```python
from build123d import *

# Parameters (mm, degrees)
SKETCH1_W           = 200
SKETCH1_H           = 150
BOSS_EXTRUDE1_DEPTH = 4
FILLET1_R           = 2
FILLET2_R           = 2
FILLET3_R           = 2
FILLET4_R           = 2
SKETCH2_W           = 8
SKETCH2_H           = 30
BOSS_EXTRUDE2_DEPTH = 4
FILLET5_R           = 2


# Some blends are built 0.0001 mm under size
with BuildPart() as part:
    # Sketch1 → Boss-Extrude1 (new body)
    with BuildSketch(Plane(origin=(0, 0, 0), x_dir=(1, 0, 0), z_dir=(0, 1, 0))):
        with Locations((-106.41025641, 19.711538462)):
            Rectangle(SKETCH1_W, SKETCH1_H)
    extrude(amount=BOSS_EXTRUDE1_DEPTH)

    # Fillet1
    fillet1_edges = [part.edges().sort_by_distance(p)[0] for p in [
        (-206.41025641, 4, -19.711538462),
        (-106.41025641, 4, -94.711538462),
    ]]
    fillet(fillet1_edges, radius=FILLET1_R)

    # Fillet2
    fillet2_edges = [part.edges().sort_by_distance(p)[0] for p in [
        (-105.41025641, 4, 55.288461538),
        (-206.41025641, 1, 55.288461538),
        (-205.824469973, 3.414213562, 55.288461538),
    ]]
    fillet(fillet2_edges, radius=FILLET2_R)

    # Fillet3
    fillet3_edges = [part.edges().sort_by_distance(p)[0] for p in [
        (-6.41025641, 1, -94.711538462),
        (-6.41025641, 3.414213562, -94.125752024),
        (-6.41025641, 1, 55.288461538),
        (-6.41025641, 4, -19.711538462),
        (-6.41025641, 3.414213562, 54.702675101),
    ]]
    fillet(fillet3_edges, radius=FILLET3_R)

    # Fillet4
    # the kernel refuses this fillet: 2 mm, written as the material it takes off along each edge
    with BuildSketch(Plane(origin=(-204.41025641, 2, -92.711538462), x_dir=(-1, 0, 0), z_dir=(0, 0, -1))) as fillet4_piece_1_section:
        Polygon((0, 0), (FILLET4_R, 0), (FILLET4_R, FILLET4_R), (0, FILLET4_R), align=None)
    fillet4_piece_1 = extrude(amount=FILLET4_R, mode=Mode.PRIVATE)
    fillet4_piece_1 = fillet4_piece_1 - Plane(origin=(-204.41025641, 2, -92.711538462), x_dir=(0.7071067811865475, -0.7071067811865475, 0), z_dir=(0, 0, -1)) * Sphere(FILLET4_R, mode=Mode.PRIVATE)
    add(fillet4_piece_1, mode=Mode.SUBTRACT)
    with BuildSketch(Plane(origin=(-206.41025641, -5, -94.711538462), x_dir=(1, 0, 0), z_dir=(0, 1, 0))) as fillet4_piece_2:
        with BuildLine():
            CenterArc((FILLET4_R, -FILLET4_R), FILLET4_R, 90, 90)
            Line((0, -FILLET4_R), (0, 0))
            Line((0, 0), (FILLET4_R, 0))
        make_face()
    extrude(amount=7, mode=Mode.SUBTRACT)

    # Sketch2 → Boss-Extrude2 (add)
    with BuildSketch(Plane(origin=(0, 4, 0), x_dir=(1, 0, 0), z_dir=(0, 1, 0))):
        with Locations((-6.865890451, 22.549136896)):
            Rectangle(SKETCH2_W, SKETCH2_H)
    extrude(amount=-BOSS_EXTRUDE2_DEPTH)

    # Fillet5
    fillet5_edges = [part.edges().sort_by_distance(p)[0] for p in [
        (-4.638073431, 0, -37.549136896),
    ]]
    fillet(fillet5_edges, radius=FILLET5_R)
    fillet5_2_edges = [part.edges().sort_by_distance(p)[0] for p in [
        (-2.865890451, 0, -21.549136896),
    ]]
    fillet(fillet5_2_edges, radius=FILLET5_R)
    fillet5_3_edges = [part.edges().sort_by_distance(p)[0] for p in [
        (-5.638073431, 0, -7.549136896),
    ]]
    fillet(fillet5_3_edges, radius=FILLET5_R)
    fillet5_4_edges = [part.edges().sort_by_distance(p)[0] for p in [
        (-6.638073431, 4, -37.549136896),
    ]]
    fillet(fillet5_4_edges, radius=FILLET5_R - 0.0001)  # a hair under: the kernel refuses the full size


solid = part.part
```
Can you work these out from the model? Positions are in its coordinate system, mm. Give positions to 0.01 mm unless a question says otherwise; leave off trailing zeros. Loops run counter-clockwise (first coordinate to the right, second up) from the corner with the lowest first, then second, coordinate; pieces in that order, holes last. Notation, with made-up numbers: M 8.5,-16 L 66.5,-16 A9 cw 66.5,-5 Z; hole C 61.5,80 d7. An arc over 180 degrees is marked long. Answer in a Markdown table with one row per item.
1. Suppose I cut it at A-A on z = -78. Write out the boundary of the cut face in (x, y), plus the area to 3 significant figures.
Taken from the geometry:
| item | result |
|---|---|
| outline | M -206.41,0 L -6.41,0 L -6.41,2 A2 ccw -8.41,4 L -204.41,4 A2 ccw -206.41,2 Z |
| area | 798 mm² |
2. For pin 1 Ø0.6 at (y, z) = (1, 29) entering from +X; pin 2 Ø1.5 at (y, z) = (3, -62) entering from -X; pin 3 Ø1.5 at (y, z) = (3, -14) entering from +X, each with a flat end and sliding along its axis, tell me the tip position at first contact or that it passes through.
Taken from the geometry:
| item | result |
|---|---|
| pin 1 | stops at x = -6.41 |
| pin 2 | stops at x = -206.39 |
| pin 3 | stops at x = -2.88 |
3. If I drill on line 1 along X through (y, z) = (0.95, 16); line 2 along Z through (x, y) = (-28.5, 2.4); line 3 along X through (y, z) = (3.25, -31.5), over which ranges is the centre line in solid material (lowest first)?
Taken from the geometry:
| item | result |
|---|---|
| line 1 | x = -206.41 to -6.41 |
| line 2 | z = -94.67 to 55.25 |
| line 3 | x = -205.97 to -3.3 |
